```python
from build123d import *

# Parameters (mm, degrees)
F0_R     = 0.75
F1_DEPTH = 4.5
F2_W     = 3
F2_H     = 2
F3_DEPTH = 3
F4_R     = 0.5


with BuildPart() as f1:
    # F0 (on Top) → F1 (new body)
    with BuildSketch(Plane.XY):
        Polygon((-2.425, 4.175), (-4.175, 4.175), (-4.175, -4.175), (4.175, -4.175), (4.175, 4.175), (2.425, 4.175), align=None)
        with BuildLine():
            Line((-2.425, 9.25), (-2.425, 4.175))
            Line((-2.425, 4.175), (2.425, 4.175))
            Line((2.425, 4.175), (2.425, 9.25))
            ThreePointArc((2.425, 9.25), (0, 11.675), (-2.425, 9.25))
        make_face()
        with Locations((0, 9.25)):
            Circle(F0_R, mode=Mode.SUBTRACT)
    extrude(amount=F1_DEPTH)

    # F2 (on face) → F3 (cut)
    with BuildSketch(Plane.XY.offset(4.5)):
        Rectangle(F2_W, F2_H)
    extrude(amount=-F3_DEPTH, mode=Mode.SUBTRACT)

    # F4
    f4_edges = [f1.edges().sort_by_distance(p)[0] for p in [
        (0, 11.675, 0),
        (2.425, 6.7125, 0),
        (-2.425, 6.7125, 0),
        (0, 11.675, 4.5),
        (2.425, 6.7125, 4.5),
        (-2.425, 6.7125, 4.5),
    ]]
    fillet(f4_edges, radius=F4_R)


solid = f1.part
```
The listing builds one solid part. Answer for the finished solid, in the listing's coordinates (mm). A direction names the side the tool comes from. Coordinates: 2 decimals unless noted, no trailing zeros. Write each loop counter-clockwise with the first axis right and the second up, starting at its lowest first coordinate (ties: lowest second). Pieces come first, ordered by that corner, then holes. Notation, with made-up numbers: (47, 81.5) - (66, 81.5) arc R22 cw to (66, 117.5) - close; hole circle Ø11 at (-23, -16.75). An arc over 180 degrees is marked (long way). Return JSON: item names as keys, results as strings. Group by question number.
1. Straight lines are drawn through the part: L1, parallel to Y at x = 0, z = 2.25 (3 decimals); L2, parallel to Y at x = 0.5, z = 3.55 (3 decimals); L3, parallel to Y at x = -4, z = 1.45 (3 decimals). For each, find the intervals that lie inside material, in ascending order.
2. A cutting plane is placed at A-A, the plane x = 0. Determine the outline of the cut face in (y, z) (3 decimals).
3. Determine the mould class of faces 1 (the cylindrical face through (0.053, 11.674, 2.226)), 2 (the flat face through (0, 2, 4.5)), 3 (the flat face through (1.5, 0, 3)), 4 (the flat face through (4.175, 0, 2)) for opening direction X: released by +X, released by -X, zero draft, split by the parting line, or undercut.
4. Given pin 1 (1.6 mm diameter, centred on x = -0.5, y = 0, fed in from +Z); pin 2 (0.7 mm diameter, centred on x = -3, z = 1.5, fed in from +Y) (3 decimals), each flat-ended and moving along its own axis, determine where each tip first touches the part or whether it passes through.
5. Which of the six approach directions +Z, -Z, +X, -X, +Y, -Y give full straight-line access (tool end or side, diameter ignored) to faces 5 (the flat face through (0, 0, 1.5)), 6 (the flat face through (2.425, 7, 2)), 7 (the flat face through (-2.425, 7, 2))?
6. A cutting plane is placed at B-B, the plane z = 1.1. Determine the outline of the cut face in (x, y) (3 decimals).
7. A cutting plane is placed at D-D, the plane z = 4.15. Determine the outline of the cut face in (x, y) (3 decimals), plus the area to 3 significant figures.
8. A cutting plane is placed at C-C, the plane y = 0.5. Determine the outline of the cut face in (x, z) (3 decimals), plus the area to 3 significant figures.
Ans:
{
 "1": {"L1": "-4.175 to -1, 1 to 8.5, 10 to 11.675", "L2": "-4.175 to -1, 1 to 8.691, 9.809 to 11.623", "L3": "-4.175 to 4.175"},
 "2": {"outline": "(-4.175, 0) - (8.5, 0) - (8.5, 4.5) - (1, 4.5) - (1, 1.5) - (-1, 1.5) - (-1, 4.5) - (-4.175, 4.5) - close; (10, 0) - (11.175, 0) arc R0.5 ccw to (11.675, 0.5) - (11.675, 4) arc R0.5 ccw to (11.175, 4.5) - (10, 4.5) - close"},
 "3": {"face 1": "split by the parting line", "face 2": "zero draft", "face 3": "undercut", "face 4": "released by +X"},
 "4": {"pin 1": "z = 1.5", "pin 2": "y = 4.175"},
 "5": {"face 5": "+Z", "face 6": "+Z, -Z, +X, +Y", "face 7": "+Z, -Z, -X, +Y"},
 "6": {"outline": "(-4.175, -4.175) - (4.175, -4.175) - (4.175, 4.175) - (2.425, 4.175) - (2.425, 9.25) arc R2.425 ccw to (-2.425, 9.25) - (-2.425, 4.175) - (-4.175, 4.175) - close; hole circle Ø1.5 at (0, 9.25)"},
 "7": {"outline": "(-4.175, -4.175) - (4.175, -4.175) - (4.175, 4.175) - (2.402, 4.175) - (2.402, 9.25) arc R2.402 ccw to (-2.402, 9.25) - (-2.402, 4.175) - (-4.175, 4.175) - close; hole (-1.5, -1) - (1.5, -1) - (1.5, 1) - (-1.5, 1) - close; hole circle Ø1.5 at (0, 9.25)", "area": "95.4 mm²"},
 "8": {"outline": "(-4.175, 0) - (4.175, 0) - (4.175, 4.5) - (1.5, 4.5) - (1.5, 1.5) - (-1.5, 1.5) - (-1.5, 4.5) - (-4.175, 4.5) - close", "area": "28.6 mm²"}
}
